Autodesk Inventor part; units mm, degrees
ref_plane "YZ Plane" through (0, 0, 0) normal (1, 0, 0) x (0, 1, 0)
ref_plane "XZ Plane" through (0, 0, 0) normal (0, 1, 0) x (-1, 0, 0)
ref_plane "XY Plane" through (0, 0, 0) normal (0, 0, 1) x (1, 0, 0)
sketch "Sketch1" plane through (0, 0, 0) normal (0, 0, 1) x (1, 0, 0)
  line L0 (0, 0) -> (-120.65, 0)
  line L1 (-120.65, 0) -> (-120.65, -50.8)
  line L2 (-120.65, -50.8) -> (0, -50.8)
  line L3 (0, -50.8) -> (0, 0)
  circle A0 centre (-31.75, -25.4) radius 14.2875
  circle A1 centre (-13.7895, -7.4395) radius 1.5875
  circle A2 centre (-49.7105, -43.3605) radius 1.5875
  dimension "d0" = 28.575
  dimension "d1" = 25.4
  dimension "d2" = 25.4
  dimension "d3" = 50.8
  dimension "d4" = 3.175
  dimension "d5" = 3.175
  dimension "d6" = 25.4
  dimension "d7" = 31.75
  dimension "d8" = 88.9
  dimension "d9" = 17.9605
  dimension "d10" = 17.9605
extrude "Extrusion1" add sketch "Sketch1" along normal blind 3.175
sketch "Sketch2" plane through (0, 0, 3.175) normal (0, 0, 1) x (1, 0, 0)
  circle A0 centre (-107.95, -12.7) radius 3.3734
  line L0 (-120.65, 0) -> (-120.65, -50.8)
  line L1 (0, 0) -> (-120.65, 0)
  circle A1 centre (-82.55, -38.1) radius 3.3734
  line L2 (-120.65, -50.8) -> (0, -50.8)
  dimension "d13" = 6.7469
  dimension "d14" = 12.7
  dimension "d15" = 12.7
  dimension "d16" = 6.7469
  dimension "d17" = 12.7
  dimension "d18" = 38.1
extrude "Extrusion2" cut sketch "Sketch2" against normal blind 3.175
properties part number "secondaryflywheelmount"
CAD build for the part. Positions are in the model's coordinates, mm. Round coordinates to 2 decimals unless told otherwise and drop trailing zeros. Write each loop counter-clockwise with the first axis right and the second up, starting at its lowest first coordinate (ties: lowest second). Pieces come first, ordered by that corner, then holes. Notation, with made-up numbers: M 3.5,73.25 L 44.5,73.25 A22 cw 44.5,96.25 Z; hole C 58,44.5 d5. An arc over 180 degrees is marked long. Use a Markdown table: item, result. Add a question column.
1. Slice it at A-A on x = -31.75. Give the cut face in (y, z) (1 decimal).
2. Slice it at C-C on y = -38.1. Give the cut face in (x, z) (3 decimals), then the cut area to 3 significant figures.
3. Drill centre lines: probe 1 along X at (y, z) = (-13, 0.55); probe 2 along Y at (x, z) = (-82.55, 2.2); probe 3 along X at (y, z) = (-26, 2.2). Where is each one in solid material? Low to high.
4. Flat gauge pin, fed straight in: P1, Ø6, axis at x = -82.55, y = -38.1, coming from the +Z side. Where does the tip first touch, or does it go through?
5. Pull direction X, two halves, no side cores. Call faces 1 (the face through (-120.65, -25, 2)), 2 (the face through (-108.681, -15.993, 1.61)), 3 (the face through (-61, -25, 3.175)): released by +X, released by -X, zero draft, split by the parting line, or undercut.
6. Slice it at D-D on z = 2.65. Give the number of separate pieces and of enclosed holes in the cut face, then the cut area to 3 significant figures.
Reply:
| question | item | result |
|---|---|---|
| 1 | outline | M -50.8,0 L -39.7,0 L -39.7,3.2 L -50.8,3.2 Z; M -11.1,0 L 0,0 L 0,3.2 L -11.1,3.2 Z |
| 2 | outline | M -120.65,0 L -85.923,0 L -85.923,3.175 L -120.65,3.175 Z; M -79.177,0 L -38.295,0 L -38.295,3.175 L -79.177,3.175 Z; M -25.205,0 L 0,0 L 0,3.175 L -25.205,3.175 Z |
| 2 | area | 320 mm^2 |
| 3 | probe 1 | x = -120.65 to -111.31, -104.59 to -38.85, -24.65 to 0 |
| 3 | probe 2 | y = -50.8 to -41.47, -34.73 to 0 |
| 3 | probe 3 | x = -120.65 to -46.02, -17.48 to 0 |
| 4 | P1 | passes through |
| 5 | face 1 | released by -X |
| 5 | face 2 | undercut |
| 5 | face 3 | zero draft |
| 6 | separate pieces | 1 |
| 6 | enclosed holes | 5 |
| 6 | area | 5,400 mm^2 |
